Work out the finished part from the listing and answer in its coordinate system (mm). A direction names the side the tool comes from. Round coordinates to 2 decimals unless told otherwise and drop trailing zeros. Order: outer loops, then holes, each group sorted by start corner. A loop starts at its lowest first (then second) coordinate and runs counter-clockwise, first axis right, second up. Notation, with made-up numbers: (-22.75, 86) - (-11.75, 86) arc R8 ccw to (-11.75, 99) - close; hole circle Ø5 at (77, -28.5). An arc over 180 degrees is marked (long way). Put each result on its own line as item: value.
```python
from build123d import *

# Parameters (mm, degrees)
ESQUISSE1_R          = 10
BOSS_EXTRU_1_DEPTH   = 50
BOSS_EXTRU_1_2_DEPTH = 50
ESQUISSE1_3_W        = 120
ESQUISSE1_3_H        = 180
BOSS_EXTRU_2_DEPTH   = 70


with BuildPart() as part:
    # Esquisse1 → Boss.-Extru.1 (new body)
    with BuildSketch(Plane(origin=(0, 0, 0), x_dir=(1, 0, 0), z_dir=(0, 1, 0))):
        with BuildLine():
            Line((-60, -90), (-60, 90))
            Line((-60, 90), (-125, 90))
            ThreePointArc((-125, 90), (-142.67766953, 82.67766953), (-150, 65))
            Line((-150, 65), (-150, -65))
            ThreePointArc((-150, -65), (-142.67766953, -82.67766953), (-125, -90))
            Line((-125, -90), (-60, -90))
        make_face()
        with Locations(Location((-125, -65, 0), (0, 0, 270))):
            Circle(ESQUISSE1_R, mode=Mode.SUBTRACT)
        with Locations(Location((-125, 65, 0), (0, 0, 270))):
            Circle(ESQUISSE1_R, mode=Mode.SUBTRACT)
    extrude(amount=BOSS_EXTRU_1_DEPTH)



with BuildPart() as body_2:
    # Esquisse1 → Boss.-Extru.1 2 (new body)
    with BuildSketch(Plane(origin=(0, 0, 0), x_dir=(1, 0, 0), z_dir=(0, 1, 0))):
        with BuildLine():
            Line((125, 90), (60, 90))
            Line((60, 90), (60, -90))
            Line((60, -90), (125, -90))
            ThreePointArc((125, -90), (142.67766953, -82.67766953), (150, -65))
            Line((150, -65), (150, 65))
            ThreePointArc((150, 65), (142.67766953, 82.67766953), (125, 90))
        make_face()
        with Locations(Location((125, -65, 0), (0, 0, 270))):
            Circle(ESQUISSE1_R, mode=Mode.SUBTRACT)
        with Locations(Location((125, 65, 0), (0, 0, 270))):
            Circle(ESQUISSE1_R, mode=Mode.SUBTRACT)
    extrude(amount=BOSS_EXTRU_1_2_DEPTH)


with BuildPart() as part_1:
    add(part.part)

    add(body_2.part)  # Boss.-Extru.2 merges body 2
    # Esquisse1_3 → Boss.-Extru.2 (add)
    with BuildSketch(Plane(origin=(0, 0, 0), x_dir=(1, 0, 0), z_dir=(0, 1, 0))):
        Rectangle(ESQUISSE1_3_W, ESQUISSE1_3_H)
    extrude(amount=BOSS_EXTRU_2_DEPTH)


solid = part_1.part
```
1) A cutting plane is placed at D-D on x = 101.5. Write down the section's boundary in (y, z), then the cut area to 3 significant figures.
Findings below:
outline: (0, -90) - (50, -90) - (50, 90) - (0, 90) - close
area: 9,000 mm2
2) Straight lines are drawn through the part: L1, parallel to X at y = 22, z = 65; L2, parallel to X at y = 17, z = 72; L3, parallel to Z at x = 131, y = 31.5. For each, find the intervals that lie inside material, in ascending order. Write a range as from..to.
Findings below:
L1: x = -150..-135, -115..115, 135..150
L2: x = -149..-132.14, -117.86..117.86, 132.14..149
L3: z = -89.27..-73, -57..57, 73..89.27
3) A cutting plane is placed at A-A on y = 42.5. Write down the section's boundary in (x, z).
Findings below:
outline: (-150, -65) arc R25 ccw to (-125, -90) - (125, -90) arc R25 ccw to (150, -65) - (150, 65) arc R25 ccw to (125, 90) - (-125, 90) arc R25 ccw to (-150, 65) - close; hole circle Ø20 at (-125, -65); hole circle Ø20 at (-125, 65); hole circle Ø20 at (125, -65); hole circle Ø20 at (125, 65)
4) For a pull along Z with two mould halves and no side action, classify faces 1 (the cylindrical face through (142.871, 24.65, -82.482)), 2 (the cylindrical face through (131.76, 24.65, -72.37)), 3 (the cylindrical face through (142.482, 24.65, 82.871)) as pulls with the +Z half, pulls with the -Z half, needs draft (parallel to the pull), parting line crosses it, or undercut.
Findings below:
face 1: pulls with the -Z half
face 2: undercut
face 3: pulls with the +Z half
5) For faces 4 (the flat face through (-2, 27, 90)), 5 (the flat face through (60, 60, 1)), 6 (the flat face through (-60, 60, 1)), determine the directions among +Z, -Z, +X, -X, +Y, -Y from which every point of the face is accessible in a straight line to the end or side of a thin tool.
Findings below:
face 4: +Z, +X, -X, +Y, -Y
face 5: +Z, -Z, +X, +Y
face 6: +Z, -Z, -X, +Y
6) Given pin 1 Ø23 at (x, z) = (-125, -65) entering from +Y; pin 2 Ø22 at (y, z) = (62, 20.5) entering from +X; pin 3 Ø2 at (y, z) = (60, 38) entering from -X, each flat-ended and moving along its own axis, determine where each tip first touches the part or whether it passes through.
Findings below:
pin 1: stops at y = 50
pin 2: stops at x = 60
pin 3: stops at x = -60
7) A cutting plane is placed at C-C on z = -20. Write down the section's boundary in (x, y), then the cut area to 3 significant figures.
Findings below:
outline: (-150, 0) - (150, 0) - (150, 50) - (60, 50) - (60, 70) - (-60, 70) - (-60, 50) - (-150, 50) - close
area: 17,400 mm2
8) A cutting plane is placed at B-B on z = -58.5. Write down the section's boundary in (x, y), then the cut area to 3 significant figures.
Findings below:
outline: (-150, 0) - (-132.6, 0) - (-132.6, 50) - (-150, 50) - close; (-117.4, 0) - (117.4, 0) - (117.4, 50) - (60, 50) - (60, 70) - (-60, 70) - (-60, 50) - (-117.4, 50) - close; (132.6, 0) - (150, 0) - (150, 50) - (132.6, 50) - close
area: 15,900 mm2
